Geometry: final body of the model. Coordinates: model frame, mm. A direction names the side the tool comes from. Give positions to 0.01 mm unless a question says otherwise; leave off trailing zeros. Write each loop counter-clockwise with the first axis right and the second up, starting at its lowest first coordinate (ties: lowest second). Pieces come first, ordered by that corner, then holes.
Autodesk Inventor part; units mm, degrees
ref_plane "Work Plane1" through (0, 0, 3.5) normal (0, 0, 1) x (1, 0, 0)
ref_plane "YZ Plane" through (0, 0, 0) normal (1, 0, 0) x (0, 1, 0)
ref_plane "XZ Plane" through (0, 0, 0) normal (0, 1, 0) x (-1, 0, 0)
sketch "Sketch1" plane through (0, 0, 0) normal (0, 0, 1) x (1, 0, 0)
  circle A0 centre (0, 0) radius 4
  circle A1 centre (0, 0) radius 11
  dimension "d0" = 8
  dimension "d1" = 22
extrude "Extrusion1" add sketch "Sketch1" along normal blind 7
sketch "Sketch2" plane through (0, 0, 7) normal (0, 0, 1) x (1, 0, 0)
  circle A0 centre (0, 0) radius 4.5
  circle A1 centre (0, 0) radius 10
  dimension "d4" = 9
  dimension "d5" = 20
extrude "Extrusion2" cut sketch "Sketch2" against normal blind 0.25
ref_plane "Work Plane1" through (0, 0, 3.5) normal (0, 0, 1) x (1, 0, 0)
mirror "Mirror1" about plane through (0, 0, 3.5) normal (0, 0, 1) of "Extrusion2"
fillet "Fillet1" radius 0.25 4 edges at (-11, 0, 7) (-11, 0, 0) (-4, 0, 0) (-4, 0, 7)
properties part number "Ball bearing"
Item 1: Pin query (flat end, axial travel): pin 1 Ø2 at (x, y) = (7.5, 0.5) entering from -Z; pin 2 Ø6.5 at (x, y) = (0, 0) entering from -Z; pin 3 Ø2 at (y, z) = (2, 4.5) entering from +X. Return the tip coordinate at first contact, or that it passes through.
Found:
pin 1: stops at z = 0.25
pin 2: passes through
pin 3: stops at x = 10.95
Item 2: Section C-C, the plane z = 2.5. Return the cut outline in (x, y).
Found:
outline: circle Ø22 at (0, 0); hole circle Ø8 at (0, 0)
Item 3: Line query: L1, parallel to Y at x = 0, z = 2.25; L2, parallel to Y at x = 0, z = 0.1; L3, parallel to Z at x = -8.25, y = -4.75. Output: solid intervals per line, ascending.
Found:
L1: y = -11 to -4, 4 to 11
L2: y = -10.95 to -10, -4.5 to -4.05, 4.05 to 4.5, 10 to 10.95
L3: z = 0.25 to 6.75
Item 4: Reachability of faces 1 (the face through (3, -10, 0)), 2 (the face through (-4.3, -2.1, 0.25)) from +Z, -Z, +X, -X, +Y, -Y: full face, straight path, thin tool, end or side. Return the list, or none.
Found:
face 1: -Z, +X, -X, +Y, -Y
face 2: -Z
Item 5: Pull-direction query (X, two-part tool) for faces 3 (the face through (-2.38, 10.74, 3.45)), 4 (the face through (3, -10, 7)), 5 (the face through (4.3, -2.1, 6.75)); classes: +X half, -X half, draft (parallel to the pull), parting line (faces both ways), or undercut.
Found:
face 3: parting line
face 4: draft
face 5: undercut
